Read the model definition and answer for the solid it produces. Units are mm, in the model's axes. A direction names the side the tool comes from. Give positions to 0.01 mm unless a question says otherwise; leave off trailing zeros. Order: outer loops, then holes, each group sorted by start corner. A loop starts at its lowest first (then second) coordinate and runs counter-clockwise, first axis right, second up. Notation, with made-up numbers: M 0.25,53 L 51.25,53 A19 ccw 51.25,83 Z; hole C 55,10.25 d3. An arc over 180 degrees is marked long. One line per item, written item: value.
from build123d import *

# Parameters (mm, degrees)
F0_R     = 2
F0_R_2   = 0.875
F1_DEPTH = 4
F6_R     = 4
F6_R_2   = 2
F7_DEPTH = 25.4


with BuildPart() as f1:
    # F0 (on Top) → F1 (new body)
    with BuildSketch(Plane.XY):
        Circle(F0_R)
        Circle(F0_R_2, mode=Mode.SUBTRACT)
    extrude(amount=F1_DEPTH)

    # F4 (on Right) → F5 (revolve)
    with BuildSketch(Plane.YZ):
        Polygon((-1.583964, 4), (-4, 4), (-2, 0), (-1.583964, 0), align=None)
    revolve(axis=Axis((0, 0, 1.998599), (0, 0, 1)))

    # F6 (on face) → F7 (join)
    with BuildSketch(Plane.XY.offset(4)):
        Circle(F6_R)
        Circle(F6_R_2, mode=Mode.SUBTRACT)
    extrude(amount=F7_DEPTH)


solid = f1.part
1) Each of these flat-tipped pins is pushed along its axis until it touches: pin 1 Ø1.2 at (x, y) = (0, -0.5) entering from +Z; pin 2 Ø3 at (x, z) = (-2, 17) entering from +Y. Where does it stop, or does it pass through?
Reported:
pin 1: stops at z = 4
pin 2: stops at y = 3.97
2) Determine the mould class of faces 1 (the face through (0.9, 0.5, 0)), 2 (the face through (0.5, 0.9, 4)), 3 (the face through (2.3, 0.3, 0.64)) for opening direction X: +X half, -X half, draft (parallel to the pull), parting line (faces both ways), or undercut.
Reported:
face 1: draft
face 2: undercut
face 3: parting line
3) Find section C-C, the plane z = 19. Write down the section's boundary in (x, y), plus the area to 3 significant figures.
Reported:
outline: C 0,0 d8; hole C 0,0 d4
area: 37.7 mm^2
4) Consider probe 1 along Y at (x, z) = (0, 17.5); probe 2 along Y at (x, z) = (-0.5, 11.25); probe 3 along Z at (x, y) = (0, -1.25). Determine where each line is inside the solid, lowest interval first.
Reported:
probe 1: y = -4 to -2, 2 to 4
probe 2: y = -3.97 to -1.94, 1.94 to 3.97
probe 3: z = 0 to 4
5) Which of the six approach directions +Z, -Z, +X, -X, +Y, -Y give full straight-line access (tool end or side, diameter ignored) to faces 4 (the face through (0, -2, 17)), 5 (the face through (-0.867, -3.905, 16.522))?
Reported:
face 4: +Z
face 5: +Z, -Z
6) Find section A-A, the plane x = 0. Write down the section's boundary in (y, z) (3 decimals).
Reported:
outline: M -4,4 L -2,0 L -0.875,0 L -0.875,4 L -2,4 L -2,29.4 L -4,29.4 Z; M 0.875,0 L 2,0 L 4,4 L 4,29.4 L 2,29.4 L 2,4 L 0.875,4 Z
